```python
from build123d import *

# Parameters (mm, degrees)
SKETCH1_R           = 3.175
BOSS_EXTRUDE2_DEPTH = 6.35
BOSS_EXTRUDE3_DEPTH = 6.35
SKETCH3_R           = 3.175
CUT_EXTRUDE1_DEPTH  = 6.35
FILLET1_R           = 2.54


with BuildPart() as part:
    # Sketch1 → Boss-Extrude2 (new body)
    with BuildSketch(Plane.XY):
        with BuildLine():
            Line((-13.229381943, 36.614978912), (29.410930021, -26.537564946))
            ThreePointArc((29.410930021, -26.537564946), (26.846901034, -39.761671923), (13.622794056, -37.197642936))
            Line((13.622794056, -37.197642936), (-0.945979198, -15.620523785))
            Line((-0.945979198, -15.620523785), (-23.975246761, -86.039905978))
            Line((-23.975246761, -86.039905978), (-42.081609524, -80.118577791))
            Line((-42.081609524, -80.118577791), (-14.448744653, 4.37778177))
            Line((-14.448744653, 4.37778177), (-29.017517907, 25.954900921))
            ThreePointArc((-29.017517907, 25.954900921), (-26.45348892, 39.179007899), (-13.229381943, 36.614978912))
        make_face()
        with Locations((-14.213437321, 21.050847952)):
            Circle(SKETCH1_R, mode=Mode.SUBTRACT)
        with Locations((14.213437321, -21.050847952)):
            Circle(SKETCH1_R, mode=Mode.SUBTRACT)
        Circle(SKETCH1_R, mode=Mode.SUBTRACT)
        with Locations((-29.080876018, -71.008333376)):
            Circle(SKETCH1_R, mode=Mode.SUBTRACT)
        with Locations((-25.133323893, -58.937424867)):
            Circle(SKETCH1_R, mode=Mode.SUBTRACT)
        with Locations((-21.185771769, -46.866516358)):
            Circle(SKETCH1_R, mode=Mode.SUBTRACT)
        with Locations((-17.238219645, -34.79560785)):
            Circle(SKETCH1_R, mode=Mode.SUBTRACT)
    extrude(amount=BOSS_EXTRUDE2_DEPTH)

    # Sketch2 → Boss-Extrude3 (add)
    with BuildSketch(Plane(origin=(0, 0, 0), x_dir=(-1, 0, 0), z_dir=(0, 0, -1))):
        Polygon((20.370072839, -13.728580993), (42.081609524, -80.118577791), (102.436152067, -60.380817169), (80.724615383, 6.009179629), align=None)
    extrude(amount=-BOSS_EXTRUDE3_DEPTH)

    # Sketch3 → Cut-Extrude1 (cut)
    with BuildSketch(Plane(origin=(0, 0, 0), x_dir=(-1, 0, 0), z_dir=(0, 0, -1))):
        with Locations((76.268181978, -0.792959837)):
            Circle(SKETCH3_R)
        with Locations((40.055456452, -12.63561621)):
            Circle(SKETCH3_R)
        with Locations((51.898112825, -48.848341736)):
            Circle(SKETCH3_R)
        with Locations((88.110838352, -37.005685363)):
            Circle(SKETCH3_R)
        with Locations((64.083147402, -24.820650786)):
            Circle(SKETCH3_R)
    extrude(amount=-CUT_EXTRUDE1_DEPTH, mode=Mode.SUBTRACT)

    # Fillet1
    fillet1_edges = [part.edges().sort_by_distance(p)[0] for p in [
        (-0.945979198, -15.620523785, 3.175),
        (-23.975246761, -86.039905978, 3.175),
        (-14.448744653, 4.37778177, 3.175),
        (-20.370072839, -13.728580993, 3.175),
        (-80.724615383, 6.009179629, 3.175),
        (-102.436152067, -60.380817169, 3.175),
    ]]
    fillet(fillet1_edges, radius=FILLET1_R)


solid = part.part
```
Check sheet for the modelled part. Datum: model origin and axes. Units: mm. A direction names the side the tool comes from. Round coordinates to 2 decimals unless told otherwise and drop trailing zeros. Order: outer loops, then holes, each group sorted by start corner. A loop starts at its lowest first (then second) coordinate and runs counter-clockwise, first axis right, second up. Notation, with made-up numbers: M 32,48.25 L 42,48.25 A20 cw 42,78.25 Z; hole C 79.5,-32.75 d11. An arc over 180 degrees is marked long. Answer in a Markdown table with one row per item.
(1) Gauge pin test, flat ends, axial feed: pin 1 (4 mm diameter, centred on x = 0, y = 0, fed in from -Z); pin 2 (10 mm diameter, centred on x = -25.13, y = -58.94, fed in from -Z); pin 3 (2 mm diameter, centred on x = -11.5, z = 3.5, fed in from +Y); pin 4 (1 mm diameter, centred on y = -42.5, z = 2, fed in from +X). Record the tip position at first contact, or that the pin passes through.
Findings:
| item | result |
|---|---|
| pin 1 | passes through |
| pin 2 | stops at z = 0 |
| pin 3 | stops at y = 35.53 |
| pin 4 | stops at x = -9.57 |
(2) Draft check along X on faces 4 (the flat face through (-34, -35, 6.35)), 5 (the cylindrical face through (-101.5, -59.9, 3.2)), 6 (the flat face through (7.87, -28.68, 3.13)). Enter one of: +X half, -X half, draft (parallel to the pull), parting line (faces both ways), or undercut.
Findings:
| item | result |
|---|---|
| face 4 | draft |
| face 5 | -X half |
| face 6 | undercut |
(3) Section check B-B on x = -57. Record the boundary of the cut face in (y, z).
Findings:
| item | result |
|---|---|
| outline | M -75.24,0 L -1.75,0 L -1.75,6.35 L -75.24,6.35 Z |
(4) Section check C-C on x = -93. Record the boundary of the cut face in (y, z).
Findings:
| item | result |
|---|---|
| outline | M -63.47,0 L -31.53,0 L -31.53,6.35 L -63.47,6.35 Z |
(5) Set-up check for faces 1 (the flat face through (-21.984, 15.537, 3.131)), 2 (the flat face through (-17.24, -4.16, 3.13)), 3 (the flat face through (-91.721, -27.617, 3.131)): record each of +Z, -Z, +X, -X, +Y, -Y from which the full face is reachable in a straight line by a thin tool's end or side.
Findings:
| item | result |
|---|---|
| face 1 | +Z, -Z, -X |
| face 2 | +Z, -Z |
| face 3 | +Z, -Z, -X, +Y |
(6) Section check A-A on x = 0. Record the boundary of the cut face in (y, z) (3 decimals), plus the area to 3 significant figures.
Findings:
| item | result |
|---|---|
| outline | M -18.809,0 L -3.175,0 L -3.175,6.35 L -18.809,6.35 Z; M 3.175,0 L 17.022,0 L 17.022,6.35 L 3.175,6.35 Z |
| area | 187 mm^2 |
(7) Material ranges on line 1 along X through (y, z) = (-37.5, 3.75); line 2 along X through (y, z) = (-21.5, 5.25); line 3 along Y through (x, z) = (-73.5, 1.25), recorded low to high. Write a range as from..to.
Findings:
| item | result |
|---|---|
| line 1 | x = -94.95..-91.25, -84.97..-18.9, -15.57..-8.1, 13.84..29.2 |
| line 2 | x = -89.72..-2.87, 3.02..11.07, 17.36..26.01 |
| line 3 | y = -69.84..-2.35, 0.76..3.65 |
